Work out the finished part from the listing and answer in its coordinate system (mm). Face numbers are marked on the shaded views. A direction names the side the tool comes from. Coordinates: 2 decimals unless noted, no trailing zeros. Loops run counter-clockwise (first coordinate to the right, second up) from the corner with the lowest first, then second, coordinate; pieces in that order, holes last. Notation, with made-up numbers: (43, -2.75) -> (74, -2.75) arc R31 cw to (74, 33.25) -> close; hole circle Ø7 at (35, 9). An arc over 180 degrees is marked (long way). Answer as CSV lines item,"result".
```python
from build123d import *

# Parameters (mm, degrees)
SKETCH1_W           = 42
SKETCH1_H           = 42
BOSS_EXTRUDE1_DEPTH = 33
SKETCH2_R           = 1
CUT_EXTRUDE1_DEPTH  = 3.5
SKETCH3_R           = 11
BOSS_EXTRUDE2_DEPTH = 1.5
SKETCH4_R           = 2.5
BOSS_EXTRUDE3_DEPTH = 13.5
CUT_EXTRUDE2_START  = -13.5
CUT_EXTRUDE2_DEPTH  = 13.5


with BuildPart() as part:
    # Sketch1 → Boss-Extrude1 (new body)
    with BuildSketch(Plane(origin=(0, 0, 0), x_dir=(1, 0, 0), z_dir=(0, 1, 0))):
        with Locations((21, 21)):
            Rectangle(SKETCH1_W, SKETCH1_H)
    extrude(amount=BOSS_EXTRUDE1_DEPTH)

    # Sketch2 → Cut-Extrude1 (cut)
    with BuildSketch(Plane(origin=(0, 33, 0), x_dir=(1, 0, 0), z_dir=(0, 1, 0))):
        with Locations(Location((5.505, 36.495, 0), (0, 0, 270))):
            Circle(SKETCH2_R)
        with Locations(Location((36.495, 36.495, 0), (0, 0, 270))):
            Circle(SKETCH2_R)
        with Locations(Location((36.495, 5.505, 0), (0, 0, 270))):
            Circle(SKETCH2_R)
        with Locations(Location((5.505, 5.505, 0), (0, 0, 270))):
            Circle(SKETCH2_R)
    extrude(amount=-CUT_EXTRUDE1_DEPTH, mode=Mode.SUBTRACT)

    # Sketch3 → Boss-Extrude2 (add)
    with BuildSketch(Plane(origin=(0, 33, 0), x_dir=(1, 0, 0), z_dir=(0, 1, 0))):
        with Locations(Location((21, 21, 0), (0, 0, 90))):
            Circle(SKETCH3_R)
    extrude(amount=BOSS_EXTRUDE2_DEPTH)

    # Sketch4 → Boss-Extrude3 (add)
    with BuildSketch(Plane(origin=(0, 34.5, 0), x_dir=(1, 0, 0), z_dir=(0, 1, 0))):
        with Locations(Location((21, 21, 0), (0, 0, 270))):
            Circle(SKETCH4_R)
    extrude(amount=BOSS_EXTRUDE3_DEPTH)

    # Sketch5 → Cut-Extrude2 (cut)
    with BuildSketch(Plane(origin=(0, 48, 0), x_dir=(1, 0, 0), z_dir=(0, 1, 0)).offset(CUT_EXTRUDE2_START)):
        with BuildLine():
            Line((19.410943676, 22.93), (22.589056324, 22.93))
            ThreePointArc((22.589056324, 22.93), (21, 23.5), (19.410943676, 22.93))
        make_face()
    extrude(amount=CUT_EXTRUDE2_DEPTH, mode=Mode.SUBTRACT)


solid = part.part
```
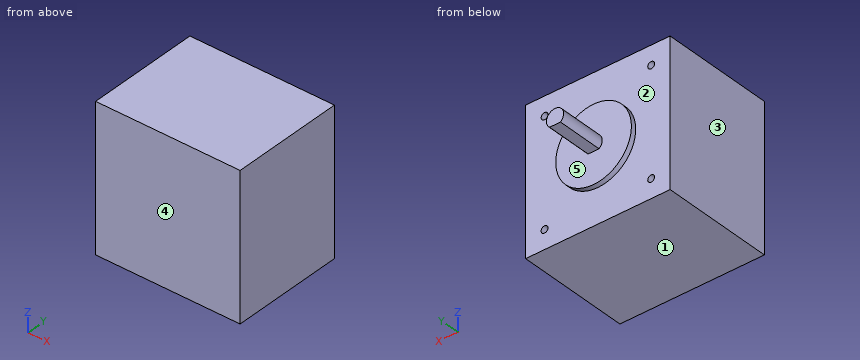
(1) Consider line 1 along Y through (x, z) = (7, -21); line 2 along Z through (x, y) = (20.5, 34); line 3 along Y through (x, z) = (21, -24). Determine where each line is inside the solid, lowest interval first.
Computed values:
line 1,"0 to 33"
line 2,"-31.99 to -10.01"
line 3,"0 to 34.5"
(2) Flat-ended cylindrical pins translate along their axes: pin 1 Ø4 at (x, z) = (16.5, -11) entering from +Y; pin 2 Ø1.6 at (x, z) = (36.5, -36.5) entering from +Y; pin 3 Ø1.5 at (x, y) = (22, 40) entering from +Z. Find the tip coordinate at first contact, or state that the pin passes through.
Computed values:
pin 1,"y = 34.5"
pin 2,"y = 29.5"
pin 3,"z = -18.51"
(3) A cutting plane is placed at B-B, the plane x = 21. Write down the section's boundary in (y, z).
Computed values:
outline,"(0, -42) -> (33, -42) -> (33, -32) -> (34.5, -32) -> (34.5, -22.93) -> (48, -22.93) -> (48, -18.5) -> (34.5, -18.5) -> (34.5, -10) -> (33, -10) -> (33, 0) -> (0, 0) -> close"
(4) A cutting plane is placed at C-C, the plane y = 37. Write down the section's boundary in (x, z), and give its area (3 significant figures).
Computed values:
outline,"(19.41, -22.93) -> (22.59, -22.93) arc R2.5 ccw (long way) to start"
area,"18.4 mm2"
(5) Which of the six approach directions +Z, -Z, +X, -X, +Y, -Y give full straight-line access (tool end or side, diameter ignored) to the marked faces 1 and 2?
Computed values:
face 1,"-Z, +X, -X, +Y, -Y"
face 2,"+Y"
(6) For a pull along Y with two mould halves and no side action, classify the marked faces 3, 4 and 5 as pulls with the +Y half, pulls with the -Y half, needs draft (parallel to the pull), parting line crosses it, or undercut.
Computed values:
face 3,"needs draft"
face 4,"pulls with the -Y half"
face 5,"pulls with the +Y half"
(7) A cutting plane is placed at D-D, the plane x = 12.5. Write down the section's boundary in (y, z).
Computed values:
outline,"(0, -42) -> (33, -42) -> (33, -27.98) -> (34.5, -27.98) -> (34.5, -14.02) -> (33, -14.02) -> (33, 0) -> (0, 0) -> close"
(8) A cutting plane is placed at A-A, the plane z = -21. Write down the section's boundary in (x, y), and give its area (3 significant figures).
Computed values:
outline,"(0, 0) -> (42, 0) -> (42, 33) -> (32, 33) -> (32, 34.5) -> (23.5, 34.5) -> (23.5, 48) -> (18.5, 48) -> (18.5, 34.5) -> (10, 34.5) -> (10, 33) -> (0, 33) -> close"
area,"1,490 mm2"
